Design review of the part built by this model. Coordinates are the model's own, in mm. A direction names the side the tool comes from. Round coordinates to 2 decimals unless told otherwise and drop trailing zeros. Write each loop counter-clockwise with the first axis right and the second up, starting at its lowest first coordinate (ties: lowest second). Pieces come first, ordered by that corner, then holes. Notation, with made-up numbers: (-17.5, 0.25) - (-0.5, 0.25) arc R23 cw to (-0.5, 12.25) - close; hole circle Ø6 at (-40, 85.5). An arc over 180 degrees is marked (long way). Use one line per item in the form item = value.
```python
from build123d import *

# Parameters (mm, degrees)
SKETCH084_W           = 10
SKETCH084_H           = 2
EXTRUDE079_DEPTH      = 5
SKETCH008_W           = 8
SKETCH008_H           = 2
EXTRUDE006_DEPTH      = 12
EXTRUDE001_DEPTH      = 9
EXTRUDE001_DEPTH_BACK = 2


with BuildPart() as extrude079:
    # Sketch084 → Extrude079 (new body)
    with BuildSketch(Plane.YZ.offset(33.5)):
        with Locations((18, 6)):
            Rectangle(SKETCH084_W, SKETCH084_H)
    extrude(amount=-EXTRUDE079_DEPTH)


with BuildPart() as compound002:
    # Sketch008 → Extrude006 (new body)
    with BuildSketch(Plane.YZ.offset(42)):
        with Locations((18, -2)):
            Rectangle(SKETCH008_W, SKETCH008_H)
    extrude(amount=-EXTRUDE006_DEPTH)

    # Compound002: union Extrude079
    add(extrude079.part)


with BuildPart() as antenna001:
    # Sketch001 → Extrude001 (new body, two sides)
    with BuildSketch(Plane.YZ.offset(33)) as extrude001_sk:
        with BuildLine():
            ThreePointArc((17.5, 3.936492), (18, 0), (18.5, 3.936492))
            Line((18.5, 5.968627), (18.5, 3.936492))
            ThreePointArc((17.5, 5.968627), (18, -2), (18.5, 5.968627))
            Line((17.5, 5.968627), (17.5, 3.936492))
        make_face()
    extrude(amount=EXTRUDE001_DEPTH)
    extrude(extrude001_sk.sketch, amount=-EXTRUDE001_DEPTH_BACK)

    # Cut003: cut Compound002
    add(compound002.part, mode=Mode.SUBTRACT)


solid = antenna001.part
```
Q1. We need section A-A on z = 2. Write out the cut boundary in (x, y), then the cut area to 3 significant figures.
Calculated:
outline = (31, 14) - (42, 14) - (42, 16) - (31, 16) - close; (31, 20) - (42, 20) - (42, 22) - (31, 22) - close
area = 44.0 mm2
Q2. To check wall thickness, follow line 1 along Y through (x, z) = (34.5, 2); line 2 along Z through (x, y) = (37.25, 18); line 3 along Y through (x, z) = (35.5, 5.5). State the ranges of each line that lie inside material, in increasing order. Write a range as from..to.
Calculated:
line_1 = 14..16, 20..22
line_2 = -1..0
line_3 = 16.06..17.5, 18.5..19.94
Q3. For P1, Ø0.6, axis at x = 39, z = 4.5, coming from the +Y side; P2, Ø2.5, axis at x = 32.5, y = 16, coming from the +Z side; P3, Ø0.8, axis at y = 19, z = 5.5, coming from the -X side, all flat-tipped, find the tip position at first contact; note any pin that passes through.
Calculated:
P1 = 21.34
P2 = 5.8
P3 = 33.5
Q4. We need section C-C on z = 3.5. Write out the cut boundary in (x, y), then the cut area to 3 significant figures.
Calculated:
outline = (31, 14.29) - (42, 14.29) - (42, 16.68) - (31, 16.68) - close; (31, 19.32) - (42, 19.32) - (42, 21.71) - (31, 21.71) - close
area = 52.5 mm2
Q5. We need section B-B on x = 33.25. Write out the cut boundary in (y, z).
Calculated:
outline = (15.35, -1) - (20.65, -1) arc R4 ccw to (20.65, 5) - (18.5, 5) - (18.5, 3.94) arc R2 cw (long way) to (17.5, 3.94) - (17.5, 5) - (15.35, 5) arc R4 ccw to start
Q6. We need section D-D on y = 18. Write out the cut boundary in (x, z).
Calculated:
outline = (31, -1) - (42, -1) - (42, 0) - (31, 0) - close
Q7. Machinability: for faces 5 (the cylindrical face through (36.577, 14.197, 3.238)), 6 (the flat face through (37, 18.5, 5)), 7 (the flat face through (32, 16, 5)), which of the approach directions +Z, -Z, +X, -X, +Y, -Y give a long, thin tool a straight path to every point of the face, cutting with its end or side? Answer none if there is none.
Calculated:
face_5 = +X, -X, -Y
face_6 = +Z, +X, -X
face_7 = +Z, -X, +Y, -Y
Q8. Draft analysis for pull direction Y (two halves, no side actions). For faces 1 (the flat face through (31, 19, 0)), 2 (the flat face through (37, 17.5, 5)), 3 (the cylindrical face through (36.58, 21.84, 3.12)), 4 (the cylindrical face through (37, 18, 0)), state which applies: released by +Y, released by -Y, zero draft, split by the parting line, or undercut.
Calculated:
face_1 = zero draft
face_2 = undercut
face_3 = released by +Y
face_4 = undercut
